The listing builds one solid part. Answer for the finished solid, in the listing's coordinates (mm). Face numbers are marked on the shaded views. Round coordinates to 2 decimals unless told otherwise and drop trailing zeros. Loops run counter-clockwise (first coordinate to the right, second up) from the corner with the lowest first, then second, coordinate; pieces in that order, holes last. Notation, with made-up numbers: (80, 71.5) - (127, 71.5) arc R19 ccw to (127, 104.5) - close; hole circle Ø11 at (8, -25.5). An arc over 180 degrees is marked (long way). Write item = value, one per line. Start each with the question number.
1) For a pull along Z with two mould halves and no side action, classify the marked faces 1, 2 and 3 as released by +Z, released by -Z, zero draft, split by the parting line, or undercut.
2) Straight lines are drawn through the part: line 1 along X through (y, z) = (1.75, 0); line 2 along Z through (x, y) = (-9, 2.25); line 3 along Z through (x, y) = (5, 6). For each, find the intervals that lie inside material, in ascending order.
3) Given pin 1 Ø4 at (y, z) = (1.5, -2.5) entering from +X; pin 2 Ø1.5 at (x, y) = (12.5, 3.5) entering from -Z; pin 3 Ø6 at (x, z) = (-2, 5.5) entering from -Y; pin 4 Ø21 at (x, z) = (3, 6.5) entering from -Y, each flat-ended and moving along its own axis, determine where each tip first touches the part or whether it passes through.
4) Section A-A, the plane x = 0 is taken. Determine the outline of the cut face in (y, z), and give its area (3 significant figures).
5) Section C-C, the plane y = 5.25 is taken. Determine the outline of the cut face in (x, z).
6) Section B-B, the plane z = 0 is taken. Determine the outline of the cut face in (x, y), and give its area (3 significant figures).
from build123d import *

# Parameters (mm, degrees)
SKETCH_1_R          = 15.2
D30_4T7_DEPTH       = 7
SKETCH_2_R          = 18.2
SKETCH_2_R_2        = 15.2
EXTRUDE_2_DEPTH     = 2
SKETCH_3_R          = 13.2
CUT_EXTRUDE_1_DEPTH = 7
CHAMFER_1_SIZE      = 0.5


with BuildPart() as part:
    # 스케치1 → D30.4t7 (new body)
    with BuildSketch(Plane(origin=(0, 0, 0), x_dir=(1, 0, 0), z_dir=(0, 1, 0))):
        with Locations(Location((0, 0, 0), (0, 0, 270))):
            Circle(SKETCH_1_R)
    extrude(amount=D30_4T7_DEPTH)

    # 스케치2 → 보스-돌출2 (add)
    # profile 1 of 3: a face of its own
    with BuildSketch(Plane(origin=(0, 7, 0), x_dir=(1, 0, 0), z_dir=(0, 1, 0))):
        with Locations(Location((0, 0, 0), (0, 0, 270))):
            Circle(SKETCH_2_R)
        with Locations(Location((0, 0, 0), (0, 0, 270))):
            Circle(SKETCH_2_R_2, mode=Mode.SUBTRACT)
    # profile 2 of 3: a face of its own
    with BuildSketch(Plane(origin=(0, 7, 0), x_dir=(1, 0, 0), z_dir=(0, 1, 0))):
        with Locations(Location((0, 0, 0), (0, 0, 270))):
            Circle(SKETCH_2_R_2)
    # profile 3 of 3: a face of its own
    with BuildSketch(Plane(origin=(0, 7, 0), x_dir=(1, 0, 0), z_dir=(0, 1, 0))):
        with Locations(Location((0, 0, 0), (0, 0, 270))):
            Circle(SKETCH_2_R_2)
    extrude(amount=EXTRUDE_2_DEPTH)

    # 스케치3 → 컷-돌출1 (cut)
    with BuildSketch(Plane.XZ):
        with Locations(Location((0, 0, 0), (0, 0, 270))):
            Circle(SKETCH_3_R)
    extrude(amount=-CUT_EXTRUDE_1_DEPTH, mode=Mode.SUBTRACT)

    # 모따기1
    chamfer_1_edges = [part.edges().sort_by_distance(p)[0] for p in [
        (0, 0, -15.2),
    ]]
    chamfer(chamfer_1_edges, length=CHAMFER_1_SIZE)


solid = part.part
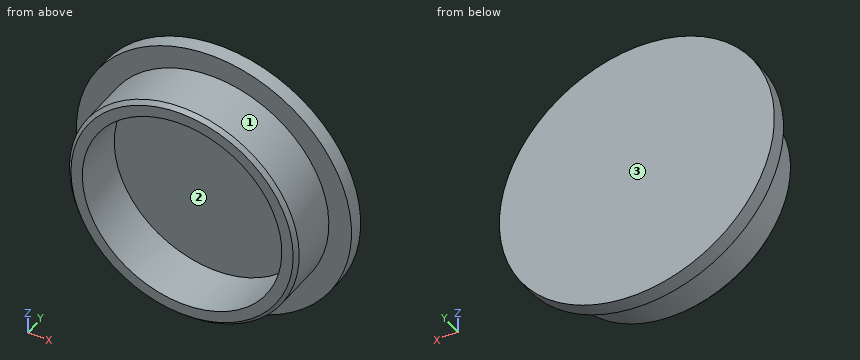
Geometry check:
q1.face_1 = split by the parting line
q1.face_2 = undercut
q1.face_3 = zero draft
q2.line_1 = -15.2 to -13.2, 13.2 to 15.2
q2.line_2 = -12.25 to -9.66, 9.66 to 12.25
q2.line_3 = -14.35 to -12.22, 12.22 to 14.35
q3.pin_1 = 15.19
q3.pin_2 = -9.64
q3.pin_3 = 7
q3.pin_4 = 0
q4.outline = (0, -14.7) - (0.5, -15.2) - (7, -15.2) - (7, -18.2) - (9, -18.2) - (9, 18.2) - (7, 18.2) - (7, 15.2) - (0.5, 15.2) - (0, 14.7) - (0, 13.2) - (7, 13.2) - (7, -13.2) - (0, -13.2) - close
q4.area = 101 mm2
q5.outline = circle Ø30.4 at (0, 0); hole circle Ø26.4 at (0, 0)
q6.outline = (-18.2, 7) - (-15.2, 7) - (-15.2, 0.5) - (-14.7, 0) - (-13.2, 0) - (-13.2, 7) - (13.2, 7) - (13.2, 0) - (14.7, 0) - (15.2, 0.5) - (15.2, 7) - (18.2, 7) - (18.2, 9) - (-18.2, 9) - close
q6.area = 101 mm2
